Here's how the part is built. I have some questions about the finished solid (model axes, mm). Coordinates: 2 decimals unless noted, no trailing zeros. Loops run counter-clockwise (first coordinate to the right, second up) from the corner with the lowest first, then second, coordinate; pieces in that order, holes last. Notation, with made-up numbers: M 41,56.5 L 93,56.5 A30 cw 93,94.5 Z; hole C 86.25,57 d10. An arc over 180 degrees is marked long. Use CSV: the item, a comma, the result in double quotes. Start each with the question number.
Q1. For pin 1 Ø2.5 at (x, y) = (-19.05, -79.375) entering from -Z (3 decimals), with a flat end and sliding along its axis, tell me the tip position at first contact or that it passes through.
Q2. If we section it at A-A (x = 0): Please give me the cut outline in (y, z) (3 decimals), and give its area (3 significant figures).
Q3. If we section it at C-C (x = -19.5): Please give me the cut outline in (y, z) (3 decimals).
Q4. If we mould it in two halves opening along Y, with no side actions, what happens to faces 1 (the cylindrical face through (-0.467, -81.476, -0.044)), 2 (the cylindrical face through (-1.59, 68.9, -0.04)), 3 (the flat face through (0, 76.2, 0)), 4 (the flat face through (0, -2, 3.175))? For each: +Y half, -Y half, draft (parallel to the pull), parting line (faces both ways), or undercut.
Q5. Please list where these lines run through material, in increasing order: probe 1 along Y at (x, z) = (0, 1.5); probe 2 along Y at (x, z) = (19.5, 2); probe 3 along X at (y, z) = (68, 0.5). Write a range as [from, to].
Q6. If we section it at B-B (x = 19.05): Please give me the cut outline in (y, z) (3 decimals), and give its area (3 significant figures).
from build123d import *

# Parameters (mm, degrees)
SKETCH1_R           = 2.15265
BOSS_EXTRUDE1_DEPTH = 3.175


with BuildPart() as part:
    # Sketch1 → Boss-Extrude1 (new, symmetric)
    with BuildSketch(Plane.XY):
        Polygon((-25.4, -76.2), (-25.4, -82.55), (25.4, -82.55), (25.4, -76.2), (25.4, 76.2), (-25.4, 76.2), align=None)
        with Locations((0, 67.4497)):
            Circle(SKETCH1_R, mode=Mode.SUBTRACT)
        with Locations((-19.05, -79.375)):
            Circle(SKETCH1_R, mode=Mode.SUBTRACT)
        with Locations((0, -79.375)):
            Circle(SKETCH1_R, mode=Mode.SUBTRACT)
        with Locations((19.05, -79.375)):
            Circle(SKETCH1_R, mode=Mode.SUBTRACT)
    extrude(amount=BOSS_EXTRUDE1_DEPTH, both=True)


solid = part.part
Results below:
1,pin 1,"through"
2,outline,"M -82.55,-3.175 L -81.528,-3.175 L -81.528,3.175 L -82.55,3.175 Z; M -77.222,-3.175 L 65.297,-3.175 L 65.297,3.175 L -77.222,3.175 Z; M 69.602,-3.175 L 76.2,-3.175 L 76.2,3.175 L 69.602,3.175 Z"
2,area,"953 mm^2"
3,outline,"M -82.55,-3.175 L -81.48,-3.175 L -81.48,3.175 L -82.55,3.175 Z; M -77.27,-3.175 L 76.2,-3.175 L 76.2,3.175 L -77.27,3.175 Z"
4,face 1,"undercut"
4,face 2,"undercut"
4,face 3,"+Y half"
4,face 4,"draft"
5,probe 1,"[-82.55, -81.53], [-77.22, 65.3], [69.6, 76.2]"
5,probe 2,"[-82.55, -81.48], [-77.27, 76.2]"
5,probe 3,"[-25.4, -2.08], [2.08, 25.4]"
6,outline,"M -82.55,-3.175 L -81.528,-3.175 L -81.528,3.175 L -82.55,3.175 Z; M -77.222,-3.175 L 76.2,-3.175 L 76.2,3.175 L -77.222,3.175 Z"
6,area,"981 mm^2"
